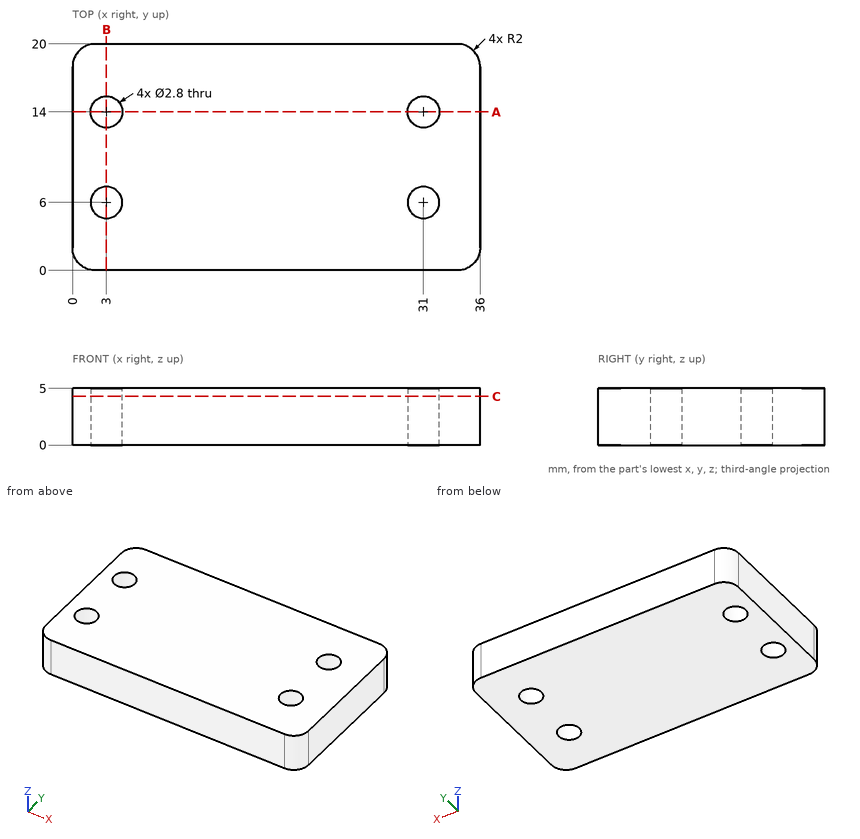
Geometry check sheet. Reference: drawing and pictorial views, mm from the part's lowest x, y, z. Coordinates: 2 decimals unless noted, no trailing zeros. Loops run counter-clockwise (first coordinate to the right, second up) from the corner with the lowest first, then second, coordinate; pieces in that order, holes last.
1) Material ranges on probe 1 along Y at (x, z) = (31, 2.25); probe 2 along X at (y, z) = (14, 2); probe 3 along X at (y, z) = (13.5, 2.85), recorded low to high.
2) Sectioned sample at A-A (y = 14). Record the boundary of the cut face in (x, z), and give its area (3 significant figures).
3) Sectioned sample at B-B (x = 3). Record the boundary of the cut face in (y, z).
4) Sectioned sample at C-C (z = 4.3). Record the boundary of the cut face in (x, y).
Check sheet entries:
1. probe 1: y = 0 to 4.6, 7.4 to 12.6, 15.4 to 20
1. probe 2: x = 0 to 1.6, 4.4 to 29.6, 32.4 to 36
1. probe 3: x = 0 to 1.69, 4.31 to 29.69, 32.31 to 36
2. outline: (0, 0) - (1.6, 0) - (1.6, 5) - (0, 5) - close; (4.4, 0) - (29.6, 0) - (29.6, 5) - (4.4, 5) - close; (32.4, 0) - (36, 0) - (36, 5) - (32.4, 5) - close
2. area: 152 mm2
3. outline: (0, 0) - (4.6, 0) - (4.6, 5) - (0, 5) - close; (7.4, 0) - (12.6, 0) - (12.6, 5) - (7.4, 5) - close; (15.4, 0) - (20, 0) - (20, 5) - (15.4, 5) - close
4. outline: (0, 2) arc R2 ccw to (2, 0) - (34, 0) arc R2 ccw to (36, 2) - (36, 18) arc R2 ccw to (34, 20) - (2, 20) arc R2 ccw to (0, 18) - close; hole circle Ø2.8 at (3, 6); hole circle Ø2.8 at (3, 14); hole circle Ø2.8 at (31, 6); hole circle Ø2.8 at (31, 14)
